Job drawing, mm, ordinate dimensions from the low corner. One solid piece. A direction names the side the tool comes from. Coordinates: 2 decimals unless noted, no trailing zeros. Write each loop counter-clockwise with the first axis right and the second up, starting at its lowest first coordinate (ties: lowest second). Pieces come first, ordered by that corner, then holes. Notation, with made-up numbers: (1.25, 29) -> (46.25, 29) arc R30 cw to (46.25, 60) -> close; hole circle Ø1 at (-28, 58.25). An arc over 180 degrees is marked (long way). One line per question, with ' | ' between items. Start each with the question number.
Item 1: Pin check, flat tips, straight feed: pin 1 (3 mm diameter, centred on y = 19, z = 1, fed in from +X); pin 2 (1.5 mm diameter, centred on x = 4.5, z = 4.5, fed in from +Y) (1 decimal); pin 3 (1.5 mm diameter, centred on y = 18, z = 3, fed in from +X); pin 4 (3 mm diameter, centred on x = 4.76, y = 12.7, fed in from +Z). Stop position of each tip, or through.
Item 2: 3-axis set-ups, long thin cutter, end or side, ignore diameter. For the marked faces 1 and 2: which of +Z, -Z, +X, -X, +Y, -Y reach the whole face in a straight line?
Item 3: Saw through at D-D (x = 5.75). List the corners of the cut face in (y, z).
Item 4: Probe probe 1 along X at (y, z) = (11.5, 3.5) (1 decimal); probe 2 along Y at (x, z) = (12.7, 2.5) (1 decimal); probe 3 along X at (y, z) = (12.5, 3.25). List the from-to ranges inside material, lowest first. Write a range as [from, to].
Item 5: Saw through at A-A (y = 12.7). Count the separate pieces of the cut face and the enclosed holes in it.
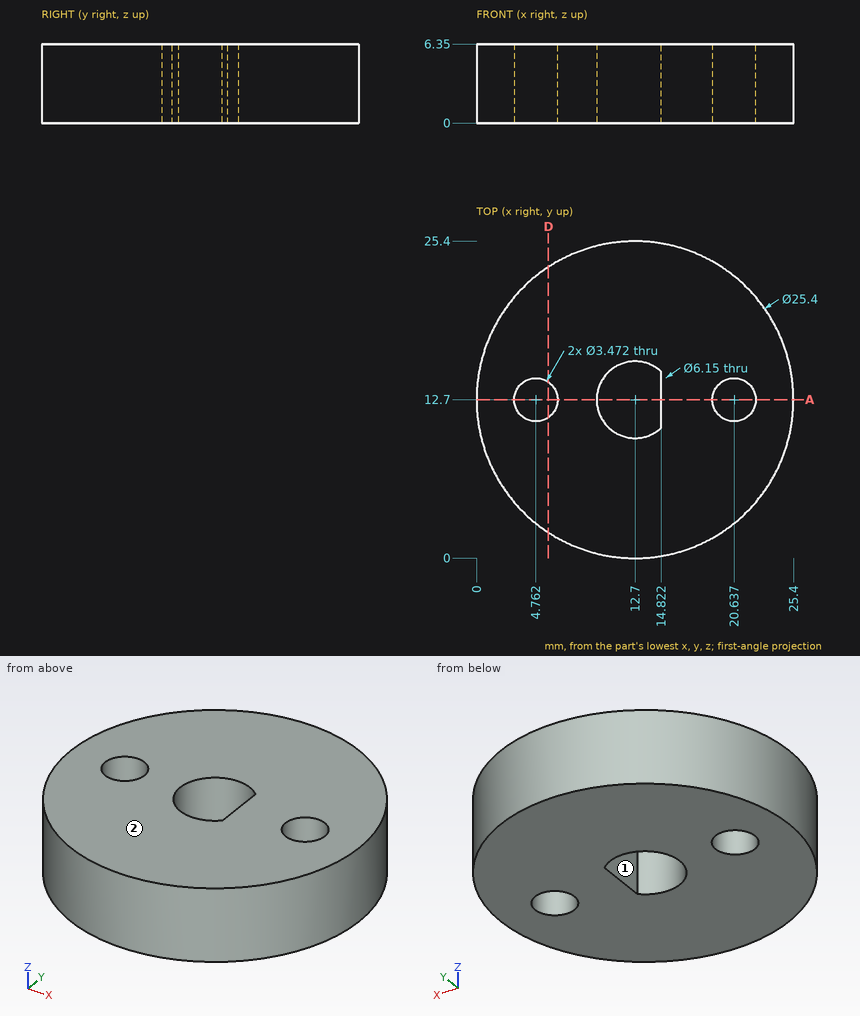
From the geometry:
1) pin 1: x = 24.46 | pin 2: y = 23 | pin 3: x = 24.56 | pin 4: through
2) face 1: +Z, -Z | face 2: +Z, +X, -X, +Y, -Y
3) outline: (2.07, 0) -> (11.27, 0) -> (11.27, 6.35) -> (2.07, 6.35) -> close; (14.13, 0) -> (23.33, 0) -> (23.33, 6.35) -> (14.13, 6.35) -> close
4) probe 1: [0.1, 3.5], [6, 9.9], [14.8, 19.4], [21.9, 25.3] | probe 2: [0, 9.6], [15.8, 25.4] | probe 3: [0, 3.04], [6.49, 9.63], [14.82, 18.91], [22.36, 25.4]
5) separate pieces: 4 | enclosed holes: 0
